```python
from build123d import *

# Parameters (mm, degrees)
F0_R     = 1.7272
F0_R_2   = 3.96875
F0_R_3   = 6.35
F0_R_4   = 8.221183
F1_DEPTH = 3.175


with BuildPart() as f1:
    # F0 (on Top) → F1 (new body)
    with BuildSketch(Plane.XY):
        with BuildLine():
            Line((-475.378193, 31.75), (-513.228467, 23.231407))
            ThreePointArc((-513.228467, 23.231407), (-531.812151, 0.128904), (-513.479674, -23.17344))
            Line((-513.479674, -23.17344), (-474.818103, -32.315493))
            Line((-474.818103, -32.315493), (-468.468103, -32.315493))
            Line((-468.468103, -32.315493), (-468.468103, -29.140493))
            Line((-468.468103, -29.140493), (-38.411718, -29.140493))
            Line((-38.411718, -29.140493), (-38.411718, -32.315493))
            Line((-38.411718, -32.315493), (-32.061718, -32.315493))
            Line((-32.061718, -32.315493), (6.126706, -21.36385))
            ThreePointArc((6.126706, -21.36385), (22.224151, 0.194294), (5.752253, 21.467701))
            Line((5.752253, 21.467701), (-32.621807, 31.75))
            Line((-32.621807, 31.75), (-38.971807, 31.75))
            Line((-38.971807, 31.75), (-38.971807, 28.575))
            Line((-38.971807, 28.575), (-469.028193, 28.575))
            Line((-469.028193, 28.575), (-469.028193, 31.75))
            Line((-469.028193, 31.75), (-475.378193, 31.75))
        make_face()
        with Locations((-454.180603, -24.377993)):
            Circle(F0_R, mode=Mode.SUBTRACT)
        with Locations((-520.909118, -12.909118)):
            Circle(F0_R, mode=Mode.SUBTRACT)
        with Locations((-495.090882, -12.909118)):
            Circle(F0_R_2, mode=Mode.SUBTRACT)
        with Locations((-52.699218, -24.377993)):
            Circle(F0_R, mode=Mode.SUBTRACT)
        with Locations((-11.786586, -11.786586)):
            Circle(F0_R_2, mode=Mode.SUBTRACT)
        with Locations((11.786586, -11.786586)):
            Circle(F0_R, mode=Mode.SUBTRACT)
        with Locations((-508, 0)):
            Circle(F0_R_3, mode=Mode.SUBTRACT)
        with Locations((-520.909118, 12.909118)):
            Circle(F0_R_2, mode=Mode.SUBTRACT)
        with Locations((-495.090882, 12.909118)):
            Circle(F0_R, mode=Mode.SUBTRACT)
        with Locations((-454.740693, 23.8125)):
            Circle(F0_R, mode=Mode.SUBTRACT)
        with Locations((-50.8, 0)):
            Circle(F0_R_4, mode=Mode.SUBTRACT)
        Circle(F0_R_3, mode=Mode.SUBTRACT)
        with Locations((-11.786586, 11.786586)):
            Circle(F0_R, mode=Mode.SUBTRACT)
        with Locations((11.786586, 11.786586)):
            Circle(F0_R_2, mode=Mode.SUBTRACT)
        with Locations((-53.259307, 23.8125)):
            Circle(F0_R, mode=Mode.SUBTRACT)
    extrude(amount=F1_DEPTH)


solid = f1.part
```
Could you check a few things on this model? Use its own coordinates, in mm. Coordinates: 2 decimals unless noted, no trailing zeros. Write each loop counter-clockwise with the first axis right and the second up, starting at its lowest first coordinate (ties: lowest second). Pieces come first, ordered by that corner, then holes. Notation, with made-up numbers: (56.25, 69) -> (73.25, 69) arc R21 cw to (73.25, 91) -> close; hole circle Ø2 at (12, -8). An arc over 180 degrees is marked (long way). Write item = value, one per line. Start each with the question number.
(1) Will these pins go through, and if not, where does the flat tip stop? pin 1 (4 mm diameter, centred on x = -52.7, y = -24.38, fed in from -Z); pin 2 (3 mm diameter, centred on x = -454.74, y = 23.81, fed in from -Z); pin 3 (1 mm diameter, centred on y = -17.5, z = 2, fed in from -X); pin 4 (1.5 mm diameter, centred on y = 2, z = 0.5, fed in from -X).
(2) I want a section at D-D (x = 0). Please give me the cut outline in (y, z) (3 decimals).
(3) I want a section at B-B (x = -508). Please give me the cut outline in (y, z) (3 decimals).
(4) I need wall thicknesses on line 1 (X direction, y = -1, z = 2.75); line 2 (Y direction, x = -94, z = 0.35) (1 decimal); line 3 (Y direction, x = -50.8, z = 1) (1 decimal). Which ranges of each line are inside material? Lowest first, please. Write a range as [from, to].
(5) We'd pull the mould along Y, two halves only. Please class faces 1 (the face through (-494.04, 27.55, 1.57)), 2 (the face through (-531.806, 0.577, 1.565)), 3 (the face through (-513.04, -3.86, 1.57)): released by +Y, released by -Y, zero draft, split by the parting line, or undercut.
(6) I want a section at A-A (y = 0). Give the number of separate pieces and of enclosed holes in the cut face, plus the area to 3 significant figures.
Result set:
q1.pin_1 = 0
q1.pin_2 = through
q1.pin_3 = -524.67
q1.pin_4 = -531.78
q2.outline = (-23.121, 0) -> (-6.35, 0) -> (-6.35, 3.175) -> (-23.121, 3.175) -> close; (6.35, 0) -> (23.009, 0) -> (23.009, 3.175) -> (6.35, 3.175) -> close
q3.outline = (-24.469, 0) -> (-6.35, 0) -> (-6.35, 3.175) -> (-24.469, 3.175) -> close; (6.35, 0) -> (24.408, 0) -> (24.408, 3.175) -> (6.35, 3.175) -> close
q4.line_1 = [-531.79, -514.27], [-501.73, -58.96], [-42.64, -6.27], [6.27, 22.2]
q4.line_2 = [-29.1, 28.6]
q4.line_3 = [-29.1, -8.2], [8.2, 28.6]
q5.face_1 = released by +Y
q5.face_2 = split by the parting line
q5.face_3 = undercut
q6.separate_pieces = 4
q6.enclosed_holes = 0
q6.area = 1,630 mm2
